For this review, take the finished solid that the model builds, in its own axes (mm). A direction names the side the tool comes from. Give positions to 0.01 mm unless a question says otherwise; leave off trailing zeros. Write each loop counter-clockwise with the first axis right and the second up, starting at its lowest first coordinate (ties: lowest second). Pieces come first, ordered by that corner, then holes. Notation, with made-up numbers: M -34,23.5 L -26,23.5 A15 cw -26,35.5 Z; hole C 66,-4.5 d5. An arc over 180 degrees is marked long. Write item = value, one per line.
Autodesk Inventor part; units mm, degrees
ref_plane "YZ Plane" through (0, 0, 0) normal (1, 0, 0) x (0, 1, 0)
ref_plane "XZ Plane" through (0, 0, 0) normal (0, 1, 0) x (-1, 0, 0)
ref_plane "XY Plane" through (0, 0, 0) normal (0, 0, 1) x (1, 0, 0)
sketch "スケッチ1" plane through (0, 0, 0) normal (1, 0, 0) x (0, 1, 0)
  line L0 (0, 0) -> (6.25, 0) construction
  line L1 (6.25, 0) -> (6.25, 2) construction
  line L2 (6.25, 2) -> (15, 2)
  line L3 (15, 2) -> (15, 10)
  line L4 (15, 10) -> (6.25, 10)
  line L5 (6.25, 10) -> (6.25, 2)
  line L6 (0, -2) -> (0, 12)
  dimension "d0" = 6.25
  dimension "d4" = 8.75
  dimension "d5" = 8
revolve "回転1" add sketch "スケッチ1" angle 180 about axis through (0, 0, -10) along (0, 0, 1)
sketch "スケッチ2" plane through (0, 6.25, 10) normal (0, 0, 1) x (1, 0, 0)
  line L0 (0, 8.75) -> (0, 2.75) construction
  line L1 (0, 0) -> (0, 8.75)
  line L2 (0, 2.75) -> (-4, 2.75) construction
  line L3 (-4, 2.75) -> (-12.5738, 2.75)
  line L4 (-12.5738, 2.75) -> (-12.5738, 9.025)
  line L5 (-12.5738, 9.025) -> (-4, 9.025)
  line L6 (-4, 9.025) -> (-4, 2.75)
  point P0 (0, -6.25)
  dimension "d7" = 6
  dimension "d8" = 4
extrude "押し出し1" cut sketch "スケッチ2" against normal through all
sketch "スケッチ4" plane through (0, -15, 2) normal (1, 0, 0) x (0, 0, -1)
  line L0 (-8, 0) -> (0, 0)
  line L1 (0, 0) -> (0, 8.75)
  point P0 (2, 15)
  point P1 (-4, 3)
  dimension "d20" = 3
  dimension "d28" = 4
hole "穴2" at (0, -12, 6) direction (-1, 0, 0) diameter 2.459 end through all
fillet "フィレット2" radius 1 5 edges at (-4, 14.4568, 6) (-4, 9, 6) (-12, 9, 6) (0, 6.25, 6) (0, -6.25, 6)
sketch "スケッチ6" plane through (-4, 10, 10) normal (-1, 0, 0) x (0, 0, 1)
  line L0 (-8, 0) -> (-8, 3.6748)
  line L1 (-8, -1) -> (0, -1)
  point P0 (-10, -10)
  point P1 (-4, 2)
  dimension "d40" = 4
  dimension "d41" = 3
hole "穴4" at (-4, 12, 6) direction (1, 0, 0) diameter 2.459 end through all
properties part number "clamp-ring" material "ステンレス鋼"
1. Machinability: for faces 5 (the face through (0, 10, 6)), 6 (the face through (-0.24, 6.53, 5.94)), 7 (the face through (-4, 11, 7)), which of the approach directions +Z, -Z, +X, -X, +Y, -Y give a long, thin tool a straight path to every point of the face, cutting with its end or side? Answer none if there is none.
Responses:
face_5 = +Z, -Z, +X, +Y, -Y
face_6 = +Z, -Z, +X
face_7 = +Z, -Z, -X, +Y
2. We need section B-B, the plane x = -5.75. Write out the cut boundary in (y, z).
Responses:
outline = M -13.85,2 L -2.45,2 L -2.45,10 L -13.85,10 Z; M 2.45,2 L 9,2 L 9,10 L 2.45,10 Z; hole C -12,6 d2.46
3. We need section C-C, the plane z = 3.25. Write out the cut boundary in (x, y).
Responses:
outline = M -12.31,8.57 A15 ccw 0,-15 L 0,-7.18 A1 ccw -0.86,-6.19 A6.25 cw -0.86,6.19 A1 ccw 0,7.18 L 0,15 A15 ccw -3.21,14.65 A1 ccw -4,13.67 L -4,10 A1 cw -5,9 L -11.49,9 A1 ccw Z
4. We need section A-A, the plane y = -12. Write out the cut boundary in (x, z), then the cut area to 3 significant figures.
Responses:
outline = M -9,2 L 0,2 L 0,4.77 L -9,4.77 Z; M -9,7.23 L 0,7.23 L 0,10 L -9,10 Z
area = 49.9 mm2
5. For line 1 along Z through (x, y) = (-7.5, -12); line 2 along Y through (x, z) = (-4.5, 6); line 3 along Y through (x, z) = (-2, 4), list the stretches that pass through material, from the lowest coordinate up. Write a range as from..to.
Responses:
line_1 = 2..4.77, 7.23..10
line_2 = -14.31..-13.23, -10.77..-4.34, 4.34..9.13
line_3 = -14.87..-5.92, 5.92..14.87
6. The part is to be moulded in two halves that separate along Z. For faces 1 (the face through (-8, 0, 2)), 2 (the face through (-8, 0, 10)), 3 (the face through (-4.13, -10.8, 6.27)), 4 (the face through (0, -10, 6)), say which applies: +Z half, -Z half, draft (parallel to the pull), parting line (faces both ways), or undercut.
Responses:
face_1 = -Z half
face_2 = +Z half
face_3 = undercut
face_4 = draft
7. Insertion check: P1, Ø3, axis at x = -8.5, z = 8, coming from the -Y side; P2, Ø3, axis at y = -12, z = 6, coming from the -X side; P3, Ø4, axis at y = 11.5, z = 4.5, coming from the -X side; P4, Ø5, axis at x = -13, y = 9, coming from the +Z side. Each pin has a flat end and moves straight along its axis. Give the tip position at first contact, or say it passes through.
Responses:
P1 = -13.27
P2 = -10.71
P3 = -4.13
P4 = 10
8. We need section D-D, the plane z = 6. Write out the cut boundary in (x, y), then the cut area to 3 significant figures.
Responses:
outline = M -12.31,8.57 A15 ccw -10.44,-10.77 L 0,-10.77 L 0,-7.18 A1 ccw -0.86,-6.19 A6.25 cw -0.86,6.19 A1 ccw 0,7.18 L 0,10.77 L -4,10.77 L -4,10 A1 cw -5,9 L -11.49,9 A1 ccw Z; M -7.07,-13.23 A15 ccw 0,-15 L 0,-13.23 Z; M -4,13.23 L 0,13.23 L 0,15 A15 ccw -3.21,14.65 A1 ccw -4,13.67 Z
area = 233 mm2
